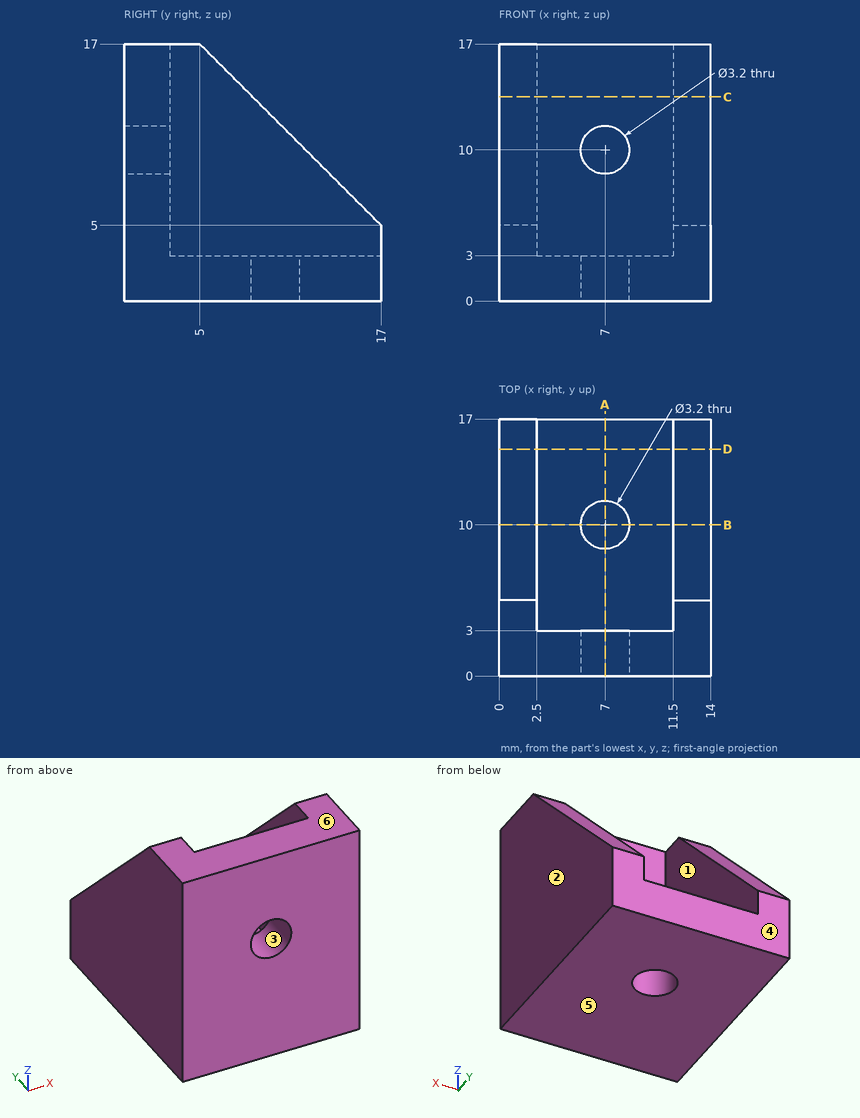
Part print with two shaded views. Sizes in mm from the minimum x, y, z corner. A direction names the side the tool comes from. Round coordinates to 2 decimals unless told otherwise and drop trailing zeros. Loops run counter-clockwise (first coordinate to the right, second up) from the corner with the lowest first, then second, coordinate; pieces in that order, holes last. Notation, with made-up numbers: (69.25, -8) - (91.25, -8) arc R27 ccw to (91.25, 22) - close; hole circle Ø10 at (-16, 42.5). An arc over 180 degrees is marked (long way). Answer as a JSON object with one key per item and string values.
Item 1: Band-saw the part on A-A on x = 7. List the corners of the cut face in (y, z), plus the area to 3 significant figures.
Output:
{"outline": "(0, 0) - (8.4, 0) - (8.4, 3) - (3, 3) - (3, 8.4) - (0, 8.4) - close; (0, 11.6) - (3, 11.6) - (3, 17) - (0, 17) - close; (11.6, 0) - (17, 0) - (17, 3) - (11.6, 3) - close", "area": "73.8 mm2"}
Item 2: Band-saw the part on D-D on y = 15. List the corners of the cut face in (x, z).
Output:
{"outline": "(0, 0) - (14, 0) - (14, 7) - (11.5, 7) - (11.5, 3) - (2.5, 3) - (2.5, 7) - (0, 7) - close"}
Item 3: Wall check: L1, parallel to X at y = 1, z = 10; L2, parallel to X at y = 7.25, z = 3.25; L3, parallel to Y at x = 7, z = 0.75. Give the ranges that are in metal, low to high.
Output:
{"L1": "0 to 5.4, 8.6 to 14", "L2": "0 to 2.5, 11.5 to 14", "L3": "0 to 8.4, 11.6 to 17"}
Item 4: Tool access for the marked faces 1 and 2: list every direction of +Z, -Z, +X, -X, +Y, -Y with a clear straight run to the whole face (end or side of a thin tool).
Output:
{"face 1": "+Z, +Y", "face 2": "+Z, -Z, +X, +Y, -Y"}
Item 5: Band-saw the part on B-B on y = 10. List the corners of the cut face in (x, z).
Output:
{"outline": "(0, 0) - (5.4, 0) - (5.4, 3) - (2.5, 3) - (2.5, 12) - (0, 12) - close; (8.6, 0) - (14, 0) - (14, 12) - (11.5, 12) - (11.5, 3) - (8.6, 3) - close"}
Item 6: Band-saw the part on C-C on z = 13.5. List the corners of the cut face in (x, y).
Output:
{"outline": "(0, 0) - (14, 0) - (14, 8.5) - (11.5, 8.5) - (11.5, 3) - (2.5, 3) - (2.5, 8.5) - (0, 8.5) - close"}
Item 7: Pull direction Z, two halves, no side cores. Call the marked faces 3, 4, 5 and 6: pulls with the +Z half, pulls with the -Z half, needs draft (parallel to the pull), parting line crosses it, or undercut.
Output:
{"face 3": "undercut", "face 4": "needs draft", "face 5": "pulls with the -Z half", "face 6": "pulls with the +Z half"}
Item 8: Pin check, flat tips, straight feed: pin 1 (1.9 mm diameter, centred on x = 7, z = 10, fed in from -Y); pin 2 (7 mm diameter, centred on x = 7, y = 12, fed in from +Z). Stop position of each tip, or through.
Output:
{"pin 1": "through", "pin 2": "z = 3"}
